Here's the drawing with two shaded views (mm, measured from the low corner). I have some questions. Round coordinates to 2 decimals unless told otherwise and drop trailing zeros. Order: outer loops, then holes, each group sorted by start corner. A loop starts at its lowest first (then second) coordinate and runs counter-clockwise, first axis right, second up. Notation, with made-up numbers: M 18.5,-16 L 28.5,-16 A29 ccw 28.5,18 Z; hole C 32,-2.5 d8. An arc over 180 degrees is marked long. One line per question, with ' | ' between items.
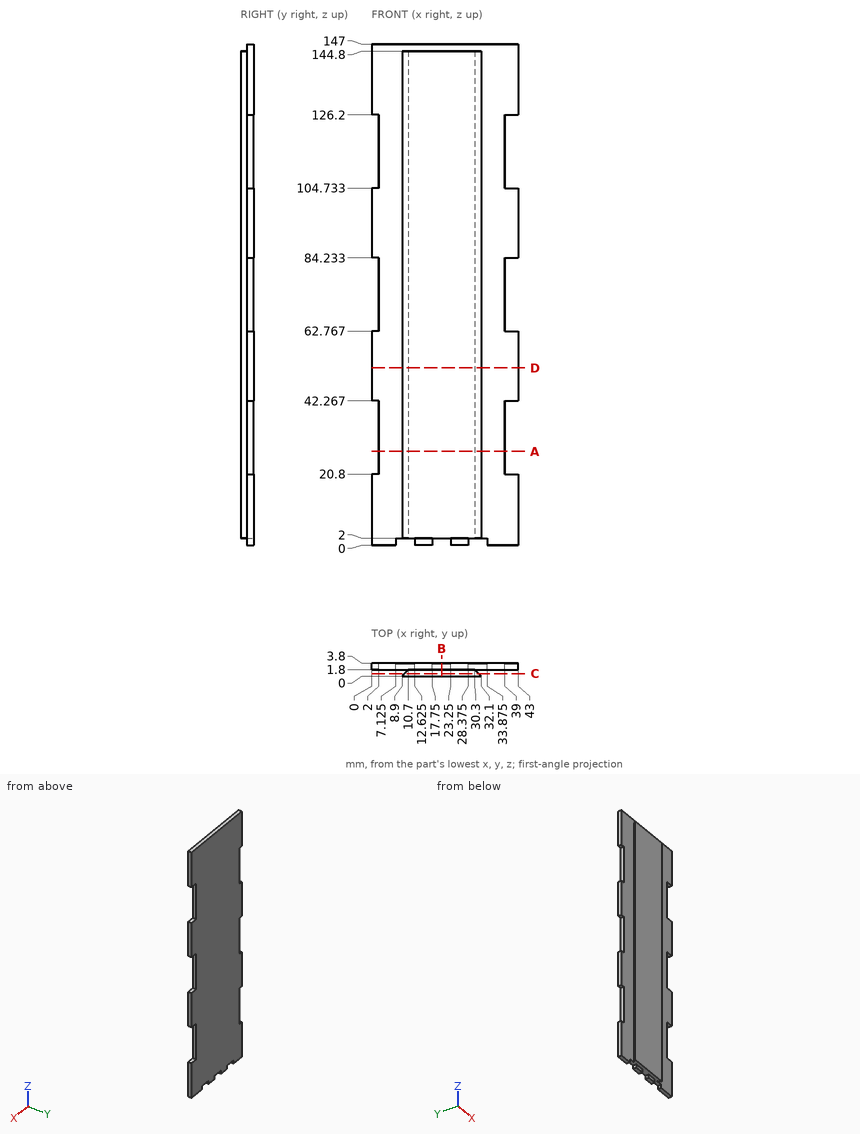
(1) If we section it at B-B on x = 20.5: Please give me the cut outline in (y, z).
Final values:
outline: M 0,2 L 3.8,2 L 3.8,147 L 1.8,147 L 1.8,144.8 L 0,144.8 Z
(2) Please list where these lines run through material, in increasing order: probe 1 along Z at (x, y) = (41, 3.3); probe 2 along Z at (x, y) = (26.5, 1.4); probe 3 along Y at (x, z) = (40, 50). Write a range as [from, to].
Final values:
probe 1: [0, 20.8], [42.27, 62.77], [84.23, 104.73], [126.2, 147] | probe 2: [2, 144.8] | probe 3: [1.8, 3.8]
(3) If we section it at D-D on z = 52: Please give me the cut outline in (x, y).
Final values:
outline: M 0,1.8 L 10.7,1.8 L 8.9,0 L 32.1,0 L 30.3,1.8 L 43,1.8 L 43,3.8 L 0,3.8 Z
(4) Will these pins go through, and if not, where does the flat tip stop? pin 1 Ø1 at (y, z) = (2.5, 35) entering from +X; pin 2 Ø2 at (y, z) = (0.5, 102.5) entering from -X; pin 3 Ø0.6 at (x, z) = (15, 1.5) entering from -Y.
Final values:
pin 1: x = 39 | pin 2: x = 8.9 | pin 3: y = 1.8
(5) If we section it at C-C on y = 0.7: Please give me the cut outline in (x, z), plus the area to 3 significant figures.
Final values:
outline: M 9.6,2 L 31.4,2 L 31.4,144.8 L 9.6,144.8 Z | area: 3,110 mm^2
(6) If we section it at A-A on z = 27.5: Please give me the cut outline in (x, y).
Final values:
outline: M 2,1.8 L 10.7,1.8 L 8.9,0 L 32.1,0 L 30.3,1.8 L 39,1.8 L 39,3.8 L 2,3.8 Z
